from build123d import *

# Parameters (mm, degrees)
SKETCH1_R           = 25
SKETCH1_R_2         = 24
BOSS_EXTRUDE1_DEPTH = 90
SKETCH2_R           = 25
SKETCH2_R_2         = 5
SKETCH2_R_3         = 1.6
BOSS_EXTRUDE2_DEPTH = 3
SKETCH3_R           = 3
CUT_EXTRUDE1_DEPTH  = 1.5
SKETCH4_R           = 1.7
SKETCH4_R_2         = 24
BOSS_EXTRUDE3_DEPTH = 4


with BuildPart() as part:
    # Sketch1 → Boss-Extrude1 (new body)
    with BuildSketch(Plane(origin=(0, 0, 0), x_dir=(0, 1, 0), z_dir=(0, 0, 1))):
        with Locations(Location((0, 0, 0), (0, 0, 90))):
            Circle(SKETCH1_R)
        with Locations(Location((0, 0, 0), (0, 0, 90))):
            Circle(SKETCH1_R_2, mode=Mode.SUBTRACT)
    extrude(amount=BOSS_EXTRUDE1_DEPTH)

    # Sketch2 → Boss-Extrude2 (add)
    with BuildSketch(Plane(origin=(90, 0, 90), x_dir=(0, 1, 0), z_dir=(0, 0, 1))):
        with Locations(Location((0, 90, 0), (0, 0, 90))):
            Circle(SKETCH2_R)
        with Locations(Location((0, 90, 0), (0, 0, 270))):
            Circle(SKETCH2_R_2, mode=Mode.SUBTRACT)
        with Locations(Location((-8.497096587, 89.777852327, 0), (0, 0, 270))):
            Circle(SKETCH2_R_3, mode=Mode.SUBTRACT)
        with Locations(Location((8.497096587, 90.222147673, 0), (0, 0, 270))):
            Circle(SKETCH2_R_3, mode=Mode.SUBTRACT)
    extrude(amount=BOSS_EXTRUDE2_DEPTH)

    # Sketch3 → Cut-Extrude1 (cut)
    with BuildSketch(Plane.XY.offset(93)):
        with Locations((-0.222147673, 8.497096587)):
            Circle(SKETCH3_R)
        with Locations((0.222147673, -8.497096587)):
            Circle(SKETCH3_R)
    extrude(amount=-CUT_EXTRUDE1_DEPTH, mode=Mode.SUBTRACT)

    # Sketch4 → Boss-Extrude3 (add)
    with BuildSketch(Plane(origin=(0, 0, 0), x_dir=(1, 0, 0), z_dir=(0, 0, -1))):
        with BuildLine():
            ThreePointArc((-8.088357722, 23.655410995), (-17.67766953, 17.67766953), (-23.655410995, 8.088357722))
            ThreePointArc((-23.655410995, 8.088357722), (-25.999890745, 4.92208801), (-29.742595978, 3.6916382))
            ThreePointArc((-29.742595978, 3.6916382), (-33.398500606, 0), (-29.742595978, -3.6916382))
            ThreePointArc((-29.742595978, -3.6916382), (-25.999890745, -4.92208801), (-23.655410995, -8.088357722))
            ThreePointArc((-23.655410995, -8.088357722), (-17.67766953, -17.67766953), (-8.088357722, -23.655410995))
            ThreePointArc((-8.088357722, -23.655410995), (-4.92208801, -25.999890745), (-3.6916382, -29.742595978))
            ThreePointArc((-3.6916382, -29.742595978), (0, -33.398500606), (3.6916382, -29.742595978))
            ThreePointArc((3.6916382, -29.742595978), (4.92208801, -25.999890745), (8.088357722, -23.655410995))
            ThreePointArc((8.088357722, -23.655410995), (17.67766953, -17.67766953), (23.655410995, -8.088357722))
            ThreePointArc((23.655410995, -8.088357722), (25.999890745, -4.92208801), (29.742595978, -3.6916382))
            ThreePointArc((29.742595978, -3.6916382), (33.398500606, 0), (29.742595978, 3.6916382))
            ThreePointArc((29.742595978, 3.6916382), (25.999890745, 4.92208801), (23.655410995, 8.088357722))
            ThreePointArc((23.655410995, 8.088357722), (17.67766953, 17.67766953), (8.088357722, 23.655410995))
            ThreePointArc((8.088357722, 23.655410995), (4.92208801, 25.999890745), (3.6916382, 29.742595978))
            ThreePointArc((3.6916382, 29.742595978), (0, 33.398500606), (-3.6916382, 29.742595978))
            ThreePointArc((-3.6916382, 29.742595978), (-4.92208801, 25.999890745), (-8.088357722, 23.655410995))
        make_face()
        with Locations(Location((0, 29.706687772, 0), (0, 0, 180))):
            Circle(SKETCH4_R, mode=Mode.SUBTRACT)
        with Locations(Location((29.706687772, 0, 0), (0, 0, 180))):
            Circle(SKETCH4_R, mode=Mode.SUBTRACT)
        with Locations(Location((0, -29.706687772, 0), (0, 0, 180))):
            Circle(SKETCH4_R, mode=Mode.SUBTRACT)
        with Locations(Location((-29.706687772, 0, 0), (0, 0, 180))):
            Circle(SKETCH4_R, mode=Mode.SUBTRACT)
        with Locations(Location((0, 0, 0), (0, 0, 180))):
            Circle(SKETCH4_R_2, mode=Mode.SUBTRACT)
    extrude(amount=-BOSS_EXTRUDE3_DEPTH)


solid = part.part
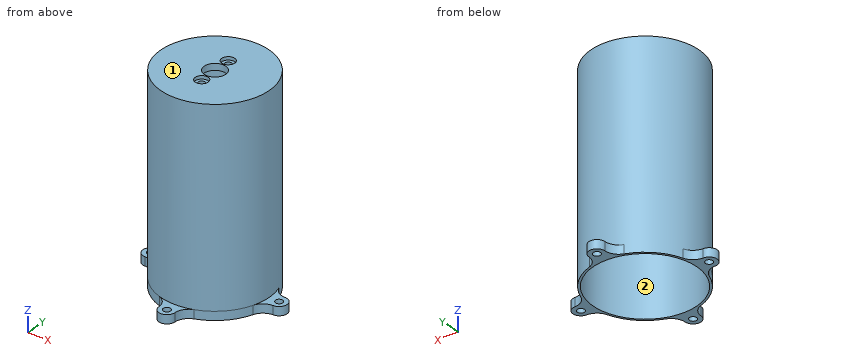
Part model, mm, in its own coordinate system. Face numbers are marked on the shaded views. Give positions to 0.01 mm unless a question says otherwise; leave off trailing zeros. Order: outer loops, then holes, each group sorted by start corner. A loop starts at its lowest first (then second) coordinate and runs counter-clockwise, first axis right, second up. Notation, with made-up numbers: (75, 36.25) - (114, 36.25) arc R31 cw to (114, 70.25) - close; hole circle Ø4 at (16, 87.25). An arc over 180 degrees is marked (long way). One line per question, with ' | ' between items.
1. Band-saw the part on B-B on x = -18. List the corners of the cut face in (y, z).
Filled in:
outline: (-17.35, 0) - (-15.87, 0) - (-15.87, 90) - (15.87, 90) - (15.87, 0) - (17.35, 0) - (17.35, 93) - (-17.35, 93) - close
2. Pull direction X, two halves, no side cores. Call the marked faces 1 and 2: +X half, -X half, draft (parallel to the pull), parting line (faces both ways), or undercut.
Filled in:
face 1: draft | face 2: undercut
3. Band-saw the part on D-D on y = 19. List the corners of the cut face in (x, z).
Filled in:
outline: (-16.25, 0) - (-14.66, 0) - (-14.66, 90) - (14.66, 90) - (14.66, 0) - (16.25, 0) - (16.25, 93) - (-16.25, 93) - close
4. Band-saw the part on C-C on z = 71.5. List the corners of the cut face in (x, y), then the cut area to 3 significant figures.
Filled in:
outline: circle Ø50 at (0, 0); hole circle Ø48 at (0, 0) | area: 154 mm²
5. Drop flat-ended pins along their axis: P1, Ø1.9, axis at x = 0.22, y = -8.5, coming from the -Z side; P2, Ø4, axis at x = 3.5, y = -11, coming from the -Z side; P3, Ø5, axis at x = 0, y = -29, coming from the +Z side; P4, Ø10, axis at y = -0.5, z = 46, coming from the -X side. Give the stop position or say it passes through.
Filled in:
P1: through | P2: z = 90 | P3: z = 4 | P4: x = -25
6. Drill centre lines: probe 1 along Y at (x, z) = (0, 92); probe 2 along X at (y, z) = (0.5, 27) (3 decimals); probe 3 along Z at (x, y) = (6.5, -5). Where is each one in solid material? Low to high.
Filled in:
probe 1: -25 to -11.49, -5.51 to -5, 5 to 5.51, 11.49 to 25 | probe 2: -24.995 to -23.995, 23.995 to 24.995 | probe 3: 90 to 93
7. Band-saw the part on A-A on y = 0. List the corners of the cut face in (x, z).
Filled in:
outline: (-33.4, 0) - (-31.41, 0) - (-31.41, 4) - (-33.4, 4) - close; (-28.01, 0) - (-24, 0) - (-24, 90) - (-5, 90) - (-5, 93) - (-25, 93) - (-25, 4) - (-28.01, 4) - close; (5, 90) - (24, 90) - (24, 0) - (28.01, 0) - (28.01, 4) - (25, 4) - (25, 93) - (5, 93) - close; (31.41, 0) - (33.4, 0) - (33.4, 4) - (31.41, 4) - close
